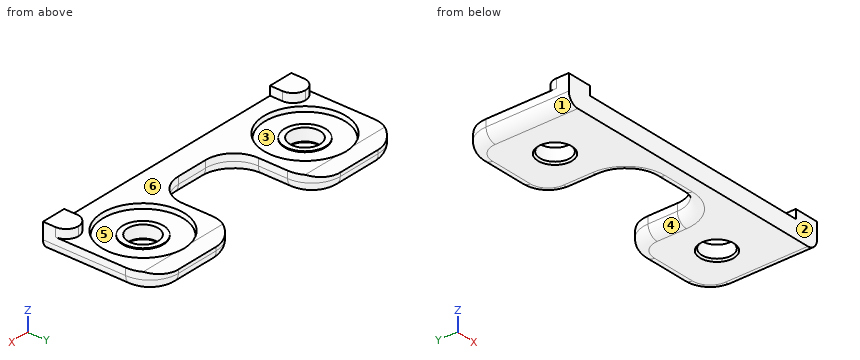
```python
from build123d import *

# Parameters (mm, degrees)
F0_W        = 7
F0_H        = 7
F0_R        = 11.25
F1_DEPTH    = 5
F0_R_2      = 5.75
F0_R_3      = 4.25
F2_DEPTH    = 3.75
F3_DEPTH    = 4
F4_DEPTH    = 7.5
F5_R        = 8
F6_T1_DEPTH = 33.2770199982
F6_T3_DEPTH = 33.2770199982
F7_R        = 3
F8_R        = 3.49999
F9_T2_ANGLE = 270
F9_T4_ANGLE = 270
F9_T6_ANGLE = 90
F9_T8_ANGLE = 90
F10_SIZE    = 0.5


# Not quite as in the source:
# - a fillet or chamfer that OpenCascade refuses, or shapes differently, is made with other operations: its cross-section is extruded or revolved along the edge and cut away or added
# - a fillet or chamfer is up to 0.001 mm smaller than in the source, because OpenCascade refuses the exact size


with BuildPart() as f1:
    # F0 (on Top) → F1 (new body)
    with BuildSketch(Plane.XY):
        with Locations((37.5, 0)):
            Rectangle(F0_W, F0_H)
        Polygon((-34, -3.5), (34, -3.5), (34, 3.5), (41, 3.5), (41, 27.75), (12.5, 27.75), (12.5, 3.5), (-12.5, 3.5), (-12.5, 27.75), (-41, 27.75), (-41, 3.5), (-34, 3.5), align=None)
        with Locations((-26.75, 12.5)):
            Circle(F0_R, mode=Mode.SUBTRACT)
        with Locations((26.75, 12.5)):
            Circle(F0_R, mode=Mode.SUBTRACT)
        with Locations((-37.5, 0)):
            Rectangle(F0_W, F0_H)
    extrude(amount=F1_DEPTH)

    # F0 (on Top) → F2 (join)
    with BuildSketch(Plane.XY):
        with Locations((-26.75, 12.5)):
            Circle(F0_R)
        with Locations((-26.75, 12.5)):
            Circle(F0_R_2, mode=Mode.SUBTRACT)
        with Locations((-26.75, 12.5)):
            Circle(F0_R_2)
        with Locations((-26.75, 12.5)):
            Circle(F0_R_3, mode=Mode.SUBTRACT)
        with Locations((26.75, 12.5)):
            Circle(F0_R)
        with Locations((26.75, 12.5)):
            Circle(F0_R_2, mode=Mode.SUBTRACT)
        with Locations((26.75, 12.5)):
            Circle(F0_R_2)
        with Locations((26.75, 12.5)):
            Circle(F0_R_3, mode=Mode.SUBTRACT)
    extrude(amount=F2_DEPTH)

    # F0 (on Top) → F3 (join)
    with BuildSketch(Plane.XY):
        with Locations((-26.75, 12.5)):
            Circle(F0_R_2)
        with Locations((-26.75, 12.5)):
            Circle(F0_R_3, mode=Mode.SUBTRACT)
        with Locations((26.75, 12.5)):
            Circle(F0_R_2)
        with Locations((26.75, 12.5)):
            Circle(F0_R_3, mode=Mode.SUBTRACT)
    extrude(amount=F3_DEPTH)

    # F0 (on Top) → F4 (join)
    with BuildSketch(Plane.XY):
        with Locations((-37.5, 0)):
            Rectangle(F0_W, F0_H)
        with Locations((37.5, 0)):
            Rectangle(F0_W, F0_H)
    extrude(amount=F4_DEPTH)

    # F5
    f5_edges = [f1.edges().sort_by_distance(p)[0] for p in [
        (-12.5, 3.5, 2.5),
        (12.5, 3.5, 2.5),
        (12.5, 27.75, 2.5),
        (41, 27.75, 2.5),
        (-41, 27.75, 2.5),
        (-12.5, 27.75, 2.5),
    ]]
    fillet(f5_edges, radius=F5_R)

    # F6: chamfer of 1 x 4 on 2 edges, made by hand

    # F6_s2 → F6_t1 (cut)
    with BuildSketch(Plane.YZ.offset(-43.3885099991)):
        Polygon((23.75, 5), (27.75, 4), (27.75, 5), align=None)
    extrude(amount=F6_T1_DEPTH, mode=Mode.SUBTRACT)

    # F6_s4 → F6_t3 (cut)
    with BuildSketch(Plane.YZ.offset(10.1114900009)):
        Polygon((23.75, 5), (27.75, 4), (27.75, 5), align=None)
    extrude(amount=F6_T3_DEPTH, mode=Mode.SUBTRACT)

    # F7
    f7_edges = [f1.edges().sort_by_distance(p)[0] for p in [
        (-26.75, 27.75, 0),
        (41, 8.125, 0),
        (38.656854, 25.406854, 0),
        (26.75, 27.75, 0),
        (-41, 8.125, 0),
        (14.843146, 25.406854, 0),
        (-38.656854, 25.406854, 0),
        (12.5, 15.625, 0),
        (10.156854, 5.843146, 0),
        (-14.843146, 25.406854, 0),
        (0, 3.5, 0),
        (-12.5, 15.625, 0),
        (-10.156854, 5.843146, 0),
    ]]
    fillet(f7_edges, radius=F7_R)

    # F8 (radius 3.5 in the source; OpenCascade refuses exactly that, so slightly less here)
    f8_edges = [f1.edges().sort_by_distance(p)[0] for p in [
        (-34, 3.5, 6.25),
        (-41, 3.5, 6.25),
        (34, 3.5, 6.25),
        (41, 3.5, 6.25),
    ]]
    fillet(f8_edges, radius=F8_R)

    # F9: chamfer of 1.25 x 0.25 on 4 edges, made by hand

    # F9_s1 → F9_t2 (revolve, cut)
    with BuildSketch(Plane.YZ.offset(-26.75)):
        Polygon((24, 5), (23.75, 3.75), (23.75, 5), align=None)
    revolve(axis=Axis((-26.75, 12.5, 5), (0, 0, 1)), revolution_arc=F9_T2_ANGLE, mode=Mode.SUBTRACT)

    # F9_s3 → F9_t4 (revolve, cut)
    with BuildSketch(Plane.YZ.offset(26.75)):
        Polygon((24, 5), (23.75, 3.75), (23.75, 5), align=None)
    revolve(axis=Axis((26.75, 12.5, 5), (0, 0, 1)), revolution_arc=F9_T4_ANGLE, mode=Mode.SUBTRACT)

    # F9_s5 → F9_t6 (revolve, cut)
    with BuildSketch(Plane.XZ.offset(-12.5)):
        Polygon((-15.25, 5), (-15.5, 3.75), (-15.5, 5), align=None)
    revolve(axis=Axis((-26.75, 12.5, 5), (0, 0, 1)), revolution_arc=F9_T6_ANGLE, mode=Mode.SUBTRACT)

    # F9_s7 → F9_t8 (revolve, cut)
    with BuildSketch(Plane.XZ.offset(-12.5)):
        Polygon((38.25, 5), (38, 3.75), (38, 5), align=None)
    revolve(axis=Axis((26.75, 12.5, 5), (0, 0, 1)), revolution_arc=F9_T8_ANGLE, mode=Mode.SUBTRACT)

    # F10
    f10_edges = [f1.edges().sort_by_distance(p)[0] for p in [
        (22.5, 12.5, 0),
        (-31, 12.5, 0),
    ]]
    chamfer(f10_edges, length=F10_SIZE)


solid = f1.part
```
Geometry: final body of the model. Coordinates: model frame, mm. Face numbers are marked on the shaded views. A direction names the side the tool comes from. Coordinates: 2 decimals unless noted, no trailing zeros. Order: outer loops, then holes, each group sorted by start corner. A loop starts at its lowest first (then second) coordinate and runs counter-clockwise, first axis right, second up. Notation, with made-up numbers: (26, 12) - (55, 12) arc R19 cw to (55, 23) - close; hole circle Ø4 at (18, 69.25). An arc over 180 degrees is marked (long way). Return JSON: item names as keys, results as strings. Group by question number.
1. Cut plane B-B (x = 26.75). Output: boundary loops of the cut face in (y, z), plus the area to 3 significant figures.
2. Pin query (flat end, axial travel): pin 1 (10 mm diameter, centred on x = -26.75, y = 12.5, fed in from +Z); pin 2 (1 mm diameter, centred on x = -31.5, z = 1.5, fed in from +Y); pin 3 (1 mm diameter, centred on x = 0, z = 4, fed in from +Y). Return the tip coordinate at first contact, or that it passes through.
3. Material intervals for line 1 along Y through (x, z) = (26.75, 3.1); line 2 along X through (y, z) = (10, 3); line 3 along X through (y, z) = (13, 2.5), sorted ascending. Write a range as [from, to].
4. Set-up query: the marked faces 4, 5 and 6. Return all of +Z, -Z, +X, -X, +Y, -Y with unobstructed straight access to the full face (end or side cutting, diameter ignored); none if empty.
5. Cut plane C-C (y = 12.5). Count the separate pieces of the cut face and the enclosed holes in it, plus the area to 3 significant figures.
6. Pull-direction query (Y, two-part tool) for the marked faces 1, 2 and 3; classes: pulls with the +Y half, pulls with the -Y half, needs draft (parallel to the pull), parting line crosses it, or undercut.
7. Cut plane D-D (z = 1.75). Output: boundary loops of the cut face in (x, y).
Resolved:
{
 "1": {"outline": "(-3.5, 0) - (7.75, 0) - (8.25, 0.5) - (8.25, 4) - (6.75, 4) - (6.75, 3.75) - (1.25, 3.75) - (1, 5) - (-3.5, 5) - close; (16.75, 0.5) - (17.25, 0) - (24.75, 0) arc R3 ccw to (27.75, 3) - (27.75, 4) - (23.99, 4.94) - (23.75, 3.75) - (18.25, 3.75) - (18.25, 4) - (16.75, 4) - close", "area": "92.5 mm²"},
 "2": {"pin 1": "stops at z = 4", "pin 2": "stops at y = 27.58", "pin 3": "stops at y = 3.5"},
 "3": {"line 1": "y = [-3.5, 8.25], [16.75, 27.75]", "line 2": "x = [-41, -30.19], [-23.31, -12.36], [12.36, 23.31], [30.19, 41]", "line 3": "x = [-40.96, -30.97], [-22.53, -12.54], [12.54, 22.53], [30.97, 40.96]"},
 "4": {"face 4": "-Z, +Y", "face 5": "+Z", "face 6": "+Z, +Y"},
 "5": {"separate pieces": "4", "enclosed holes": "0", "area": "158 mm²"},
 "6": {"face 1": "needs draft", "face 2": "pulls with the -Y half", "face 3": "undercut"},
 "7": {"outline": "(-40.73, -3.5) - (40.73, -3.5) - (40.73, 19.75) arc R7.73 ccw to (33, 27.48) - (20.5, 27.48) arc R7.73 ccw to (12.77, 19.75) - (12.77, 11.5) arc R8.27 cw to (4.5, 3.23) - (-4.5, 3.23) arc R8.27 cw to (-12.77, 11.5) - (-12.77, 19.75) arc R7.73 ccw to (-20.5, 27.48) - (-33, 27.48) arc R7.73 ccw to (-40.73, 19.75) - close; hole circle Ø8.5 at (-26.75, 12.5); hole circle Ø8.5 at (26.75, 12.5)"}
}
